from build123d import *

# Parameters (mm, degrees)
SKETCH1_W           = 345
SKETCH1_H           = 750
SKETCH1_R           = 2.2
SKETCH1_R_2         = 2.1
SKETCH1_W_2         = 260
SKETCH1_H_2         = 570
BOSS_EXTRUDE1_DEPTH = 1
SKETCH2_R           = 1.6
CUT_EXTRUDE1_DEPTH  = 1
SKETCH3_R           = 1.6
CUT_EXTRUDE2_DEPTH  = 1


with BuildPart() as part:
    # Sketch1 → Boss-Extrude1 (new body)
    with BuildSketch(Plane.XY):
        with Locations((-501.064232917, -457.603531907)):
            Rectangle(SKETCH1_W, SKETCH1_H)
        with Locations((-432.564232917, -809.582438144)):
            Circle(SKETCH1_R, mode=Mode.SUBTRACT)
        with Locations((-432.564232917, -745.582438144)):
            Circle(SKETCH1_R, mode=Mode.SUBTRACT)
        with Locations((-546.564232917, -735.582438144)):
            Circle(SKETCH1_R, mode=Mode.SUBTRACT)
        with Locations((-569.564232917, -809.582438144)):
            Circle(SKETCH1_R, mode=Mode.SUBTRACT)
        with Locations((-501.064232917, -90.603531907)):
            Circle(SKETCH1_R_2, mode=Mode.SUBTRACT)
        with Locations((-616.064232917, -90.603531907)):
            Circle(SKETCH1_R_2, mode=Mode.SUBTRACT)
        with Locations((-386.064232917, -90.603531907)):
            Circle(SKETCH1_R_2, mode=Mode.SUBTRACT)
        with Locations((-616.01978091, -720.603531907)):
            Circle(SKETCH1_R_2, mode=Mode.SUBTRACT)
        with Locations((-501.01978091, -720.603531907)):
            Circle(SKETCH1_R_2, mode=Mode.SUBTRACT)
        with Locations((-386.01978091, -720.603531907)):
            Circle(SKETCH1_R_2, mode=Mode.SUBTRACT)
        with Locations((-386.064232917, -824.603531907)):
            Circle(SKETCH1_R_2, mode=Mode.SUBTRACT)
        with Locations((-501.064232917, -824.603531907)):
            Circle(SKETCH1_R_2, mode=Mode.SUBTRACT)
        with Locations((-616.064232917, -824.603531907)):
            Circle(SKETCH1_R_2, mode=Mode.SUBTRACT)
        with Locations((-501.01978091, -427.603531907)):
            Rectangle(SKETCH1_W_2, SKETCH1_H_2, mode=Mode.SUBTRACT)
        with BuildLine():
            Line((-436.704232917, -798.532438144), (-436.704232917, -746.832438144))
            ThreePointArc((-436.704232917, -746.832438144), (-439.633165105, -739.761370332), (-446.704232917, -736.832438144))
            Line((-446.704232917, -736.832438144), (-506.704232917, -736.832438144))
            Line((-506.704232917, -736.832438144), (-512.270368826, -742.582438144))
            Line((-512.270368826, -742.582438144), (-561.204232917, -742.582438144))
            ThreePointArc((-561.204232917, -742.582438144), (-568.275300729, -745.511370332), (-571.204232917, -752.582438144))
            Line((-571.204232917, -752.582438144), (-571.204232917, -792.782438144))
            ThreePointArc((-571.204232917, -792.782438144), (-568.275300729, -799.853505955), (-561.204232917, -802.782438144))
            Line((-561.204232917, -802.782438144), (-512.270368826, -802.782438144))
            Line((-512.270368826, -802.782438144), (-506.704232917, -808.532438144))
            Line((-506.704232917, -808.532438144), (-446.704232917, -808.532438144))
            ThreePointArc((-446.704232917, -808.532438144), (-439.633165105, -805.603505955), (-436.704232917, -798.532438144))
        make_face(mode=Mode.SUBTRACT)
    extrude(amount=BOSS_EXTRUDE1_DEPTH)

    # Sketch2 → Cut-Extrude1 (cut)
    with BuildSketch(Plane.XY.offset(1)):
        with Locations((-669.634232917, -97.603531907)):
            Circle(SKETCH2_R)
        with Locations((-669.634232917, -817.603531907)):
            Circle(SKETCH2_R)
        with Locations((-669.634232917, -757.603531907)):
            Circle(SKETCH2_R)
        with Locations((-669.634232917, -697.603531907)):
            Circle(SKETCH2_R)
        with Locations((-669.634232917, -637.603531907)):
            Circle(SKETCH2_R)
        with Locations((-669.634232917, -577.603531907)):
            Circle(SKETCH2_R)
        with Locations((-669.634232917, -517.603531907)):
            Circle(SKETCH2_R)
        with Locations((-669.634232917, -457.603531907)):
            Circle(SKETCH2_R)
        with Locations((-669.634232917, -397.603531907)):
            Circle(SKETCH2_R)
        with Locations((-669.634232917, -337.603531907)):
            Circle(SKETCH2_R)
        with Locations((-669.634232917, -277.603531907)):
            Circle(SKETCH2_R)
        with Locations((-669.634232917, -217.603531907)):
            Circle(SKETCH2_R)
        with Locations((-669.634232917, -157.603531907)):
            Circle(SKETCH2_R)
    extrude(amount=-CUT_EXTRUDE1_DEPTH, mode=Mode.SUBTRACT)

    # Sketch3 → Cut-Extrude2 (cut)
    with BuildSketch(Plane.XY.offset(1)):
        with Locations((-332.514232917, -97.603531907)):
            Circle(SKETCH3_R)
        with Locations((-332.514232917, -817.603531907)):
            Circle(SKETCH3_R)
        with Locations((-332.514232917, -757.603531907)):
            Circle(SKETCH3_R)
        with Locations((-332.514232917, -697.603531907)):
            Circle(SKETCH3_R)
        with Locations((-332.514232917, -637.603531907)):
            Circle(SKETCH3_R)
        with Locations((-332.514232917, -577.603531907)):
            Circle(SKETCH3_R)
        with Locations((-332.514232917, -517.603531907)):
            Circle(SKETCH3_R)
        with Locations((-332.514232917, -457.603531907)):
            Circle(SKETCH3_R)
        with Locations((-332.514232917, -397.603531907)):
            Circle(SKETCH3_R)
        with Locations((-332.514232917, -337.603531907)):
            Circle(SKETCH3_R)
        with Locations((-332.514232917, -277.603531907)):
            Circle(SKETCH3_R)
        with Locations((-332.514232917, -217.603531907)):
            Circle(SKETCH3_R)
        with Locations((-332.514232917, -157.603531907)):
            Circle(SKETCH3_R)
    extrude(amount=-CUT_EXTRUDE2_DEPTH, mode=Mode.SUBTRACT)


solid = part.part
Can you work these out from the model? Positions are in its coordinate system, mm. Coordinates: 2 decimals unless noted, no trailing zeros. Loops run counter-clockwise (first coordinate to the right, second up) from the corner with the lowest first, then second, coordinate; pieces in that order, holes last. Notation, with made-up numbers: M 83,74 L 101,74 A13 ccw 101,80 Z; hole C -20,60 d6. An arc over 180 degrees is marked long. Return JSON: item names as keys, results as strings. Group by question number.
Item 1: Imagine slicing it at C-C (x = -535.5). Please give me the cut outline in (y, z), and give its area (3 significant figures).
Item 2: I'm going to push flat-ended pins straight in: pin 1 Ø5.5 at (x, y) = (-432.56, -745.58) entering from +Z; pin 2 Ø2.5 at (x, y) = (-332.51, -97.6) entering from +Z. Where does each tip first touch, or does it pass through?
Item 3: Imagine slicing it at B-B (y = -534.5). Please give me the cut outline in (x, z).
Item 4: If I drill on L1, parallel to Y at x = -471, z = 0.65; L2, parallel to X at y = -720.5, z = 0.45; L3, parallel to Y at x = -402.5, z = 0.65, over which ranges is the centre line in solid material (lowest first)? Write a range as from..to.
Item 5: Imagine slicing it at A-A (x = -606). Please give me the cut outline in (y, z), and give its area (3 significant figures).
Item 6: Imagine slicing it at D-D (x = -482.5). Please give me the cut outline in (y, z), and give its area (3 significant figures).
Verdict:
{
 "1": {"outline": "M -832.6,0 L -802.78,0 L -802.78,1 L -832.6,1 Z; M -742.58,0 L -712.6,0 L -712.6,1 L -742.58,1 Z; M -142.6,0 L -82.6,0 L -82.6,1 L -142.6,1 Z", "area": "120 mm^2"},
 "2": {"pin 1": "stops at z = 1", "pin 2": "passes through"},
 "3": {"outline": "M -673.56,0 L -631.02,0 L -631.02,1 L -673.56,1 Z; M -371.02,0 L -328.56,0 L -328.56,1 L -371.02,1 Z"},
 "4": {"L1": "y = -832.6..-808.53, -736.83..-712.6, -142.6..-82.6", "L2": "x = -673.56..-618.12, -613.92..-503.12, -498.92..-388.12, -383.92..-328.56", "L3": "y = -832.6..-712.6, -142.6..-82.6"},
 "5": {"outline": "M -832.6,0 L -712.6,0 L -712.6,1 L -832.6,1 Z; M -142.6,0 L -82.6,0 L -82.6,1 L -142.6,1 Z", "area": "180 mm^2"},
 "6": {"outline": "M -832.6,0 L -808.53,0 L -808.53,1 L -832.6,1 Z; M -736.83,0 L -712.6,0 L -712.6,1 L -736.83,1 Z; M -142.6,0 L -82.6,0 L -82.6,1 L -142.6,1 Z", "area": "108 mm^2"}
}
